from build123d import *

# Parameters (mm, degrees)
BOSS_EXTRUDE1_START = 8
SKETCH1_R           = 12
BOSS_EXTRUDE1_DEPTH = 8.34
SKETCH3_W           = 5.1
SKETCH3_H           = 5.1
CUT_EXTRUDE4_DEPTH  = 9


with BuildPart() as part:
    # Sketch1 → Boss-Extrude1 (new body)
    with BuildSketch(Plane.XY.offset(BOSS_EXTRUDE1_START)):
        Circle(SKETCH1_R)
    extrude(amount=-BOSS_EXTRUDE1_DEPTH)

    # Sketch3 → Cut-Extrude4 (cut, through all)
    with BuildSketch(Plane.XY):
        Rectangle(SKETCH3_W, SKETCH3_H)
    extrude(amount=CUT_EXTRUDE4_DEPTH, mode=Mode.SUBTRACT)


solid = part.part
Build history of the part. All positions in model axes, mm. A direction names the side the tool comes from. Round coordinates to 2 decimals unless told otherwise and drop trailing zeros. Loops run counter-clockwise (first coordinate to the right, second up) from the corner with the lowest first, then second, coordinate; pieces in that order, holes last. Notation, with made-up numbers: (-4.75, 69.25) -> (5.25, 69.25) arc R26 ccw to (5.25, 103.25) -> close; hole circle Ø8 at (14.25, 55.5). An arc over 180 degrees is marked (long way). One line per item, written item: value. Start each with the question number.
Q1. Cut at B-B on y = 0. List the corners of the cut face in (x, z).
Q2. Cut at A-A on z = 1.75. List the corners of the cut face in (x, y), plus the area to 3 significant figures.
Q3. Probe line 1 along Y through (x, z) = (0, 3.25); line 2 along Z through (x, y) = (0.5, -1.25); line 3 along Y through (x, z) = (1.5, 2.5). List the from-to ranges inside material, lowest first.
Q4. Drop flat-ended pins along their axis: pin 1 Ø1.5 at (x, z) = (-3.5, 4.5) entering from +Y; pin 2 Ø2 at (y, z) = (6.5, 0.5) entering from -X; pin 3 Ø1.5 at (y, z) = (-0.5, 3.5) entering from -X; pin 4 Ø1.5 at (x, y) = (-0.5, -0.5) entering from +Z. Give the stop position or say it passes through.
Q5. Two-plate mould, pull along Y, no slides. Class faces 3 (the face through (0, -2.55, 4)), 4 (the face through (0, 3, 8)), 5 (the face through (-11.99, 0.53, 3.89)): released by +Y, released by -Y, zero draft, split by the parting line, or undercut.
Q6. 3-axis set-ups, long thin cutter, end or side, ignore diameter. For faces 1 (the face through (-2.55, 0, 4)), 2 (the face through (0, 0, -0.34)): which of +Z, -Z, +X, -X, +Y, -Y reach the whole face in a straight line?
Q7. Cut at D-D on x = 10.5. List the corners of the cut face in (y, z), plus the area to 3 significant figures.
Computed:
1. outline: (-12, -0.34) -> (12, -0.34) -> (12, 8) -> (2.55, 8) -> (2.55, 0) -> (-2.55, 0) -> (-2.55, 8) -> (-12, 8) -> close
2. outline: circle Ø24 at (0, 0); hole (-2.55, -2.55) -> (2.55, -2.55) -> (2.55, 2.55) -> (-2.55, 2.55) -> close
2. area: 426 mm²
3. line 1: -12 to -2.55, 2.55 to 12
3. line 2: -0.34 to 0
3. line 3: -11.91 to -2.55, 2.55 to 11.91
4. pin 1: y = 11.68
4. pin 2: x = -10.67
4. pin 3: x = -12
4. pin 4: z = 0
5. face 3: undercut
5. face 4: zero draft
5. face 5: split by the parting line
6. face 1: +Z
6. face 2: -Z, +X, -X, +Y, -Y
7. outline: (-5.81, -0.34) -> (5.81, -0.34) -> (5.81, 8) -> (-5.81, 8) -> close
7. area: 96.9 mm²
